from build123d import *

# Parameters (mm, degrees)
POCKET_DEPTH = 4.5
BOX_W        = 23.25
BOX_H        = 10
BOX_DEPTH    = 10
SKETCH002_R  = 0.4
PAD_DEPTH    = 3.5
SKETCH003_W  = 0.8
SKETCH003_H  = 10
PAD001_DEPTH = 0.8


with BuildPart() as pocket:
    # Sketch → Revolution (revolve)
    with BuildSketch(Plane.XZ):
        Polygon((10, 3), (0, 3), (0, 0), (25, 0), (25, 3), (19.3, 3), (19.3, 1.5), (10, 1.5), align=None)
    revolve(axis=Axis((0, 0, 0), (1, 0, 0)))

    # Sketch001 → Pocket (cut)
    with BuildSketch(Plane(origin=(25, 0, 0), x_dir=(0, 0, 1), z_dir=(1, 0, 0))):
        with BuildLine():
            ThreePointArc((3, 1.5), (0, 4.499985), (-3, 1.5))
            Line((-3, 1.5), (3, 1.5))
        make_face()
    extrude(amount=-POCKET_DEPTH, mode=Mode.SUBTRACT)


with BuildPart() as fusion:
    # Box → Box (new body)
    with BuildSketch(Plane(origin=(-23.25, -5, -5), x_dir=(1, 0, 0), z_dir=(0, 0, 1))):
        with Locations((11.625, 5)):
            Rectangle(BOX_W, BOX_H)
    extrude(amount=BOX_DEPTH)

    # Sketch002 → Pad (new body)
    with BuildSketch(Plane(origin=(-23.25, 5, -5), x_dir=(-1, 0, 0), z_dir=(0, 1, 0))):
        with Locations((-18.25, 7.5)):
            Circle(SKETCH002_R)
        with Locations((-18.25, 5)):
            Circle(SKETCH002_R)
        with Locations((-18.25, 2.5)):
            Circle(SKETCH002_R)
        with Locations((-15.75, 7.5)):
            Circle(SKETCH002_R)
        with Locations((-15.75, 5)):
            Circle(SKETCH002_R)
        with Locations((-15.75, 2.5)):
            Circle(SKETCH002_R)
    extrude(amount=PAD_DEPTH)

    # Sketch003 → Pad001 (new body)
    with BuildSketch(Plane(origin=(0, -5, -5), x_dir=(0, 1, 0), z_dir=(1, 0, 0))):
        with Locations((9.6, 5)):
            Rectangle(SKETCH003_W, SKETCH003_H)
    extrude(amount=PAD001_DEPTH)

    # Fusion: union Pocket
    add(pocket.part)


solid = fusion.part
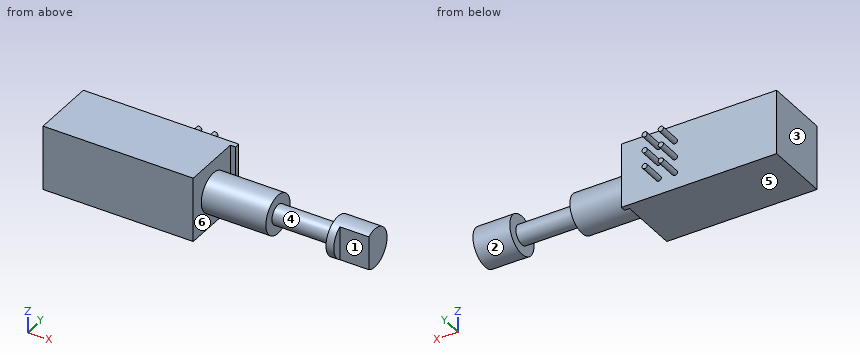
Source: CAD feature listing. Evaluate the final solid. Frame: model axes, mm. Face numbers are marked on the shaded views. A direction names the side the tool comes from. Give positions to 0.01 mm unless a question says otherwise; leave off trailing zeros. Write each loop counter-clockwise with the first axis right and the second up, starting at its lowest first coordinate (ties: lowest second). Pieces come first, ordered by that corner, then holes. Notation, with made-up numbers: M -8.75,49 L 21.25,49 A11 cw 21.25,67 Z; hole C 46,57.25 d7. An arc over 180 degrees is marked long. Return JSON: item names as keys, results as strings. Group by question number.
1) Cut plane C-C, the plane y = 0. Output: boundary loops of the cut face in (x, z), plus the area to 3 significant figures.
2) Pin query (flat end, axial travel): P1, Ø2, axis at x = 24, z = 1, coming from the -Y side; P2, Ø1, axis at x = -14, z = -3.5, coming from the +Y side; P3, Ø1, axis at y = 3.5, z = -2.5, coming from the +X side; P4, Ø5, axis at y = 7, z = -1, coming from the -X side. Return the tip coordinate at first contact, or that it passes through.
3) Cut plane D-D, the plane x = 14.5. Output: boundary loops of the cut face in (y, z), plus the area to 3 significant figures.
4) Cut plane A-A, the plane y = 6.5. Output: boundary loops of the cut face in (x, z), plus the area to 3 significant figures.
5) Set-up query: the marked faces 1, 2 and 3. Return all of +Z, -Z, +X, -X, +Y, -Y with unobstructed straight access to the full face (end or side cutting, diameter ignored); none if empty.
6) Cut plane B-B, the plane z = -3.5. Output: boundary loops of the cut face in (x, y), plus the area to 3 significant figures.
7) Material intervals for line 1 along X through (y, z) = (2.5, -1.5); line 2 along X through (y, z) = (2.5, 3.5); line 3 along Y through (x, z) = (-21, -0.75), sorted ascending. Write a range as [from, to].
8) Pull-direction query (X, two-part tool) for the marked faces 4, 5 and 6; classes: pulls with the +X half, pulls with the -X half, needs draft (parallel to the pull), parting line crosses it, or undercut.
Recorded:
{
 "1": {"outline": "M -23.25,-5 L 0,-5 L 0,-3 L 10,-3 L 10,-1.5 L 19.3,-1.5 L 19.3,-3 L 25,-3 L 25,3 L 19.3,3 L 19.3,1.5 L 10,1.5 L 10,3 L 0,3 L 0,5 L -23.25,5 Z", "area": "355 mm²"},
 "2": {"P1": "stops at y = -1.5", "P2": "stops at y = 5", "P3": "stops at x = 0", "P4": "stops at x = -23.25"},
 "3": {"outline": "C 0,0 d3", "area": "7.07 mm²"},
 "4": {"outline": "C -7.5,-2.5 d0.8; C -7.5,0 d0.8; C -7.5,2.5 d0.8; C -5,-2.5 d0.8; C -5,0 d0.8; C -5,2.5 d0.8", "area": "3.02 mm²"},
 "5": {"face 1": "+Z, -Z, +X, -Y", "face 2": "+X", "face 3": "+Z, -Z, -X, +Y, -Y"},
 "6": {"outline": "M -23.25,-5 L 0,-5 L 0,4.2 L 0.8,4.2 L 0.8,5 L -23.25,5 Z", "area": "233 mm²"},
 "7": {"line 1": "x = [-23.25, 10], [19.3, 25]", "line 2": "x = [-23.25, 0]", "line 3": "y = [-5, 5]"},
 "8": {"face 4": "undercut", "face 5": "needs draft", "face 6": "pulls with the +X half"}
}
